Input: part model. Units: mm. Frame: model coordinates. A direction names the side the tool comes from. Round coordinates to 2 decimals unless told otherwise and drop trailing zeros. Order: outer loops, then holes, each group sorted by start corner. A loop starts at its lowest first (then second) coordinate and runs counter-clockwise, first axis right, second up. Notation, with made-up numbers: (-11.75, -7) -> (42.25, -7) arc R25 cw to (42.25, 19) -> close; hole circle Ø10 at (34, 32). An arc over 180 degrees is marked (long way). Use a Markdown table: item, result.
from build123d import *

# Parameters (mm, degrees)
CHAMFER1_SIZE = 1
FILLET1_R     = 0.5


with BuildPart() as part:
    # Sketch1 → Revolve1 (revolve)
    with BuildSketch(Plane.XY):
        Polygon((24.5, 3.175), (12.5, 3.175), (12.5, 5.175), (0, 5.175), (0, 3.175), (-10, 3.175), (-10, 1.5), (24.5, 1.5), align=None)
    revolve(axis=Axis((-42.941315625, 0, 0), (1, 0, 0)))

    # Chamfer1
    chamfer1_edges = [part.edges().sort_by_distance(p)[0] for p in [
        (-10, -3.175, 0),
    ]]
    chamfer(chamfer1_edges, length=CHAMFER1_SIZE)

    # Fillet1
    fillet1_edges = [part.edges().sort_by_distance(p)[0] for p in [
        (0, -5.175, 0),
        (12.5, -5.175, 0),
    ]]
    fillet(fillet1_edges, radius=FILLET1_R)


solid = part.part
1) Draft query along Y for faces 1 (the face through (-4.56, -0.69, -3.1)), 2 (the face through (24.5, -0.7, 1.5)), 3 (the face through (7.49, -1.5, 0.07)). Return one class per face: released by +Y, released by -Y, zero draft, split by the parting line, or undercut.
Answer key:
| item | result |
|---|---|
| face 1 | split by the parting line |
| face 2 | zero draft |
| face 3 | undercut |
2) Set-up query: faces 4 (the face through (18.42, -0.69, -3.1)), 5 (the face through (6.17, -4.107, -3.149)). Return all of +Z, -Z, +X, -X, +Y, -Y with unobstructed straight access to the full face (end or side cutting, diameter ignored); none if empty.
Answer key:
| item | result |
|---|---|
| face 4 | +X |
| face 5 | +X, -X |
3) Ray query, probe 1 along Z at (x, y) = (-1, 0) (3 decimals); probe 2 along X at (y, z) = (-1.75, -3.25); probe 3 along Z at (x, y) = (7.5, 0) (3 decimals). Return the intervals inside material, ascending.
Answer key:
| item | result |
|---|---|
| probe 1 | z = -3.175 to -1.5, 1.5 to 3.175 |
| probe 2 | x = 0 to 12.5 |
| probe 3 | z = -5.175 to -1.5, 1.5 to 5.175 |
4) Cut plane A-A on y = 0. Return loops of the section in (x, z) (3 decimals).
Answer key:
| item | result |
|---|---|
| outline | (-10, -2.175) -> (-9, -3.175) -> (0, -3.175) -> (0, -4.675) arc R0.5 ccw to (0.5, -5.175) -> (12, -5.175) arc R0.5 ccw to (12.5, -4.675) -> (12.5, -3.175) -> (24.5, -3.175) -> (24.5, -1.5) -> (-10, -1.5) -> close; (-10, 1.5) -> (24.5, 1.5) -> (24.5, 3.175) -> (12.5, 3.175) -> (12.5, 4.675) arc R0.5 ccw to (12, 5.175) -> (0.5, 5.175) arc R0.5 ccw to (0, 4.675) -> (0, 3.175) -> (-9, 3.175) -> (-10, 2.175) -> close |
5) Contact query for flat-ended pins moving along their axis: P1, Ø2.5, axis at y = 0, z = 0, coming from the -X side; P2, Ø6, axis at x = 18.5, y = -2, coming from the -Z side (3 decimals); P3, Ø4, axis at x = 11.5, y = -0.5, coming from the -Z side (3 decimals); P4, Ø2, axis at x = 6, z = -2, coming from the -Y side. Output: stop coordinate, or through.
Answer key:
| item | result |
|---|---|
| P1 | passes through |
| P2 | stops at z = -3.175 |
| P3 | stops at z = -5.175 |
| P4 | stops at y = -5.08 |
6) Cut plane C-C on x = 10. Return loops of the section in (y, z) (3 decimals).
Answer key:
| item | result |
|---|---|
| outline | circle Ø10.35 at (0, 0); hole circle Ø3 at (0, 0) |
7) Cut plane D-D on x = 18. Return loops of the section in (y, z) (3 decimals).
Answer key:
| item | result |
|---|---|
| outline | circle Ø6.35 at (0, 0); hole circle Ø3 at (0, 0) |
